Build history of the part. All positions in model axes, mm. Give positions to 0.01 mm unless a question says otherwise; leave off trailing zeros. Loops run counter-clockwise (first coordinate to the right, second up) from the corner with the lowest first, then second, coordinate; pieces in that order, holes last.
1) Band-saw the part on A-A on y = 63. List the corners of the cut face in (x, z).
2) Flat gauge pins, fed straight in: P1, Ø1.5, axis at x = -37, y = 8, coming from the -Z side; P2, Ø4, axis at x = -62, z = -20, coming from the +Y side; P3, Ø6, axis at x = -60, y = 53, coming from the +Z side; P4, Ø19, axis at x = -53, z = -58, coming from the +Y side. Where does each tip first touch, or does it go through?
3) Two-plate mould, pull along X, no slides. Class faces 1 (the cylindrical face through (-8, 1, -26)), 2 (the flat face through (-40, 5, -50)), 3 (the flat face through (-39, 0, -49)): +X half, -X half, draft (parallel to the pull), parting line (faces both ways), or undercut.
4) Wall check: line 1 (X direction, y = 53.5, z = -50); line 2 (Z direction, x = -40, y = 31.5); line 3 (Z direction, x = -32, y = 29). Give the ranges that are in metal, low to high.
Autodesk Inventor part; units mm, degrees
ref_plane "YZ Plane" through (0, 0, 0) normal (1, 0, 0) x (0, 1, 0)
ref_plane "XZ Plane" through (0, 0, 0) normal (0, 1, 0) x (-1, 0, 0)
ref_plane "XY Plane" through (0, 0, 0) normal (0, 0, 1) x (1, 0, 0)
sketch "Schizzo1" plane through (0, 0, 0) normal (0, 1, 0) x (-1, 0, 0)
  circle A0 centre (40, -50) radius 40
  point P0 (0, 0)
extrude "Estrusione1" add sketch "Schizzo1" along normal blind 5
fillet "Raccordo1" radius 3 1 edges at (0, 5, -50)
sketch "Schizzo2" plane through (-40, 5, -50) normal (0, 1, 0) x (1, 0, 0)
  circle A0 centre (0, 0) radius 37
  point P0 (40, -50)
extrude "Estrusione2" add sketch "Schizzo2" along normal blind 65
fillet "Raccordo2" radius 3 2 edges at (-40, 5, -87) (-40, 5, -13)
sketch "Schizzo3" plane through (-40, 70, -50) normal (0, 1, 0) x (1, 0, 0)
  circle A0 centre (0, 0) radius 35
  point P0 (40, -50)
  dimension "d8" = 70
extrude "Estrusione3" cut sketch "Schizzo3" against normal blind 65
fillet "Raccordo3" radius 1 2 edges at (-75, 70, -50) (-77, 70, -50)
fillet "Raccordo4" radius 3 1 edges at (-75, 5, -50)
properties part number "BASE"
Findings below:
1. outline: circle Ø74 at (-40, -50); hole circle Ø70 at (-40, -50)
2. P1: stops at z = -86.93
2. P2: stops at y = 70
2. P3: stops at z = -17.14
2. P4: stops at y = 5
3. face 1: parting line
3. face 2: undercut
3. face 3: draft
4. line 1: x = -77 to -75, -5 to -3
4. line 2: z = -87 to -85, -15 to -13
4. line 3: z = -86.12 to -84.07, -15.93 to -13.88
